from build123d import *

# Parameters (mm, degrees)
F1_DEPTH = 8
F2_R     = 10
F3_R     = 5


with BuildPart() as f1:
    # F0 (on Right) → F1 (new body)
    with BuildSketch(Plane.YZ):
        Polygon((-69.120196, 185.029493), (-101.120196, 185.029493), (-101.120196, 171.029493), (-98.120196, 171.029493), (-98.120196, 175.029493), (-88.620196, 175.029493), (-88.620196, 165.029493), (30.379804, 165.029493), (30.379804, 175.029493), (39.879804, 175.029493), (39.879804, 171.029493), (42.879804, 171.029493), (42.879804, 185.029493), (10.879804, 185.029493), (10.879804, 175.029493), (2.879804, 175.029493), (2.879804, 185.029493), (-61.120196, 185.029493), (-61.120196, 175.029493), (-69.120196, 175.029493), align=None)
    extrude(amount=-F1_DEPTH)

    # F2
    f2_edges = [f1.edges().sort_by_distance(p)[0] for p in [
        (-4, -101.120196, 185.029493),
        (-4, 42.879804, 185.029493),
    ]]
    fillet(f2_edges, radius=F2_R)

    # F3
    f3_edges = [f1.edges().sort_by_distance(p)[0] for p in [
        (-4, -88.620196, 165.029493),
        (-4, 30.379804, 165.029493),
    ]]
    fillet(f3_edges, radius=F3_R)


solid = f1.part
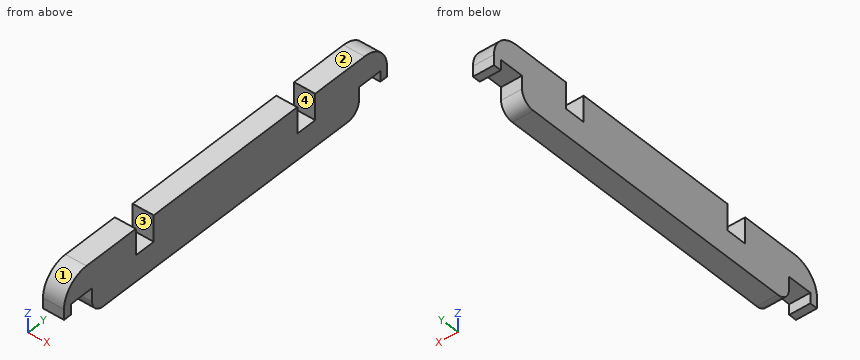
For this review, take the finished solid that the model builds, in its own axes (mm). Face numbers are marked on the shaded views. Coordinates: 2 decimals unless noted, no trailing zeros. Order: outer loops, then holes, each group sorted by start corner. A loop starts at its lowest first (then second) coordinate and runs counter-clockwise, first axis right, second up. Notation, with made-up numbers: (12.25, 30.25) -> (21.25, 30.25) arc R19 cw to (21.25, 50.25) -> close; hole circle Ø7 at (40.5, 79.25). An arc over 180 degrees is marked (long way). Return JSON: item names as keys, results as strings.
1. We need section A-A on z = 181. Write out the cut boundary in (x, y).
Answer block:
{"outline": "(-8, -99.14) -> (0, -99.14) -> (0, -69.12) -> (-8, -69.12) -> close; (-8, -61.12) -> (0, -61.12) -> (0, 2.88) -> (-8, 2.88) -> close; (-8, 10.88) -> (0, 10.88) -> (0, 40.9) -> (-8, 40.9) -> close"}
2. We need section B-B on x = -1.5. Write out the cut boundary in (y, z), and give its area (3 significant figures).
Answer block:
{"outline": "(-101.12, 171.03) -> (-98.12, 171.03) -> (-98.12, 175.03) -> (-88.62, 175.03) -> (-88.62, 170.03) arc R5 ccw to (-83.62, 165.03) -> (25.38, 165.03) arc R5 ccw to (30.38, 170.03) -> (30.38, 175.03) -> (39.88, 175.03) -> (39.88, 171.03) -> (42.88, 171.03) -> (42.88, 175.03) arc R10 ccw to (32.88, 185.03) -> (10.88, 185.03) -> (10.88, 175.03) -> (2.88, 175.03) -> (2.88, 185.03) -> (-61.12, 185.03) -> (-61.12, 175.03) -> (-69.12, 175.03) -> (-69.12, 185.03) -> (-91.12, 185.03) arc R10 ccw to (-101.12, 175.03) -> close", "area": "2,440 mm²"}
3. For line 1 (Y direction, x = -3, z = 171.25); line 2 (Y direction, x = -5, z = 182); line 3 (Z direction, x = -1.25, y = -91.5), list the stretches that pass through material, from the lowest coordinate up. Write a range as from..to.
Answer block:
{"line 1": "-101.12..-98.12, -88.62..30.38, 39.88..42.88", "line 2": "-98.29..-69.12, -61.12..2.88, 10.88..40.05", "line 3": "175.03..185.02"}
4. For pin 1 Ø6 at (y, z) = (15.5, 172) entering from +X; pin 2 Ø0.9 at (x, y) = (-5, -99.5) entering from -Z; pin 3 Ø2.5 at (x, y) = (-5, -94) entering from -Z; pin 4 Ø4 at (x, z) = (-4, 180.5) entering from -Y, all flat-tipped, find the tip position at first contact; note any pin that passes through.
Answer block:
{"pin 1": "x = 0", "pin 2": "z = 171.03", "pin 3": "z = 175.03", "pin 4": "y = -100.5"}
5. The part is to be moulded in two halves that separate along Y. For the marked faces 1, 2, 3 and 4, say which applies: +Y half, -Y half, draft (parallel to the pull), parting line (faces both ways), or undercut.
Answer block:
{"face 1": "-Y half", "face 2": "draft", "face 3": "undercut", "face 4": "undercut"}
